Here's how the part is built. I have some questions about the finished solid (model axes, mm). Coordinates: 2 decimals unless noted, no trailing zeros. Loops run counter-clockwise (first coordinate to the right, second up) from the corner with the lowest first, then second, coordinate; pieces in that order, holes last.
```python
from build123d import *

# Parameters (mm, degrees)
EXTRUDE_THIN1_DEPTH     = 301.625
SKETCH2_W               = 301.625
SKETCH2_H               = 114.3
CUT_EXTRUDE1_DEPTH      = 677.275
CUT_EXTRUDE1_DEPTH_BACK = 4.175


with BuildPart() as part:
    # Sketch1 → Extrude-Thin1 (new body)
    with BuildSketch(Plane(origin=(0, 0, 0), x_dir=(1, 0, 0), z_dir=(0, 1, 0))):
        Polygon((-339.725, -152.4), (-339.725, 152.4), (339.725, 152.4), (339.725, -152.4), (336.55, -152.4), (336.55, 149.225), (-336.55, 149.225), (-336.55, -152.4), align=None)
    extrude(amount=EXTRUDE_THIN1_DEPTH)

    # Sketch2 → Cut-Extrude1 (cut, two sides)
    with BuildSketch(Plane(origin=(-336.55, 0, 0), x_dir=(0, 0, -1), z_dir=(1, 0, 0))) as cut_extrude1_sk:
        with Locations((-1.5875, 57.15)):
            Rectangle(SKETCH2_W, SKETCH2_H)
    extrude(amount=CUT_EXTRUDE1_DEPTH, mode=Mode.SUBTRACT)
    extrude(cut_extrude1_sk.sketch, amount=-CUT_EXTRUDE1_DEPTH_BACK, mode=Mode.SUBTRACT)


solid = part.part
```
1. I want a section at D-D (y = 38). Please give me the cut outline in (x, z) (3 decimals), then the cut area to 3 significant figures.
2. I want a section at C-C (x = -196). Please give me the cut outline in (y, z) (3 decimals).
3. We'd pull the mould along X, two halves only. Please class faces 1 (the flat face through (336.55, 207, 4)), 2 (the flat face through (339.725, 182, -2)), 3 (the flat face through (-339.725, 182, 2)), 4 (the flat face through (-5, 149, -152.4)): +X half, -X half, draft (parallel to the pull), parting line (faces both ways), or undercut.
4. For pin 1 (2 mm diameter, centred on x = -213.5, y = 236.5, fed in from +Z) (3 decimals); pin 2 (3.5 mm diameter, centred on x = 337.5, z = -8.5, fed in from -Y), each with a flat end and sliding along its axis, tell me the tip position at first contact or that it passes through.
5. I want a section at A-A (z = -35.5). Please give me the cut outline in (x, y) (3 decimals).
6. I need wall thicknesses on line 1 along X through (y, z) = (268, -110) (3 decimals); line 2 along Z through (x, y) = (-267, 28.5) (3 decimals). Which ranges of each line are inside material? Lowest first, please.
7. I want a section at B-B (y = 283.5). Please give me the cut outline in (x, z) (3 decimals).
Response values:
1. outline: (-339.725, -152.4) - (339.725, -152.4) - (339.725, -149.225) - (-339.725, -149.225) - close
1. area: 2,160 mm2
2. outline: (0, -152.4) - (301.625, -152.4) - (301.625, -149.225) - (0, -149.225) - close
3. face 1: undercut
3. face 2: +X half
3. face 3: -X half
3. face 4: draft
4. pin 1: stops at z = -149.225
4. pin 2: stops at y = 114.3
5. outline: (-339.725, 114.3) - (-336.55, 114.3) - (-336.55, 301.625) - (-339.725, 301.625) - close; (336.55, 114.3) - (339.725, 114.3) - (339.725, 301.625) - (336.55, 301.625) - close
6. line 1: x = -339.725 to -336.55, 336.55 to 339.725
6. line 2: z = -152.4 to -149.225
7. outline: (-339.725, -152.4) - (339.725, -152.4) - (339.725, 152.4) - (336.55, 152.4) - (336.55, -149.225) - (-336.55, -149.225) - (-336.55, 152.4) - (-339.725, 152.4) - close
